Geometry check sheet. Reference: the model listing, model coordinates, mm. Face numbers are marked on the shaded views. A direction names the side the tool comes from. Coordinates: 2 decimals unless noted, no trailing zeros. Order: outer loops, then holes, each group sorted by start corner. A loop starts at its lowest first (then second) coordinate and runs counter-clockwise, first axis right, second up. Notation, with made-up numbers: M -24,71 L -1,71 A11 cw -1,79 Z; hole C 57.5,54 d2. An arc over 180 degrees is marked long. One line per item, written item: value. Start each with the question number.
1) Thickness scan on L1, parallel to Y at x = 0, z = 13.5; L2, parallel to X at y = 4, z = 17. Record the ranges inside material, lowest first. Write a range as from..to.
2) Go/stop test with flat-tipped pins: P1, Ø2.5, axis at x = 0, y = 0, coming from the -Z side; P2, Ø1.5, axis at x = 3.5, y = -1.5, coming from the -Z side; P3, Ø1.5, axis at y = -1.5, z = 31.5, coming from the -X side; P4, Ø3.5, axis at x = 0, y = 0, coming from the +Z side. Record where each tip stops, or that it passes through.
3) Sectioned sample at A-A, the plane x = 0. Enter the section's corners in (y, z).
4) Sectioned sample at D-D, the plane x = -3.5. Enter the section's corners in (y, z), then the cut area to 3 significant figures.
5) Draft check along Y on the marked faces 3, 4 and 5. Enter one of: pulls with the +Y half, pulls with the -Y half, needs draft (parallel to the pull), parting line crosses it, or undercut.
6) Sectioned sample at C-C, the plane z = 28. Enter the section's corners in (x, y), then the cut area to 3 significant figures.
7) Access from +Z, -Z, +X, -X, +Y, -Y to the whole of each face (thin tool, end or side, straight path). Record for the marked faces 1 and 2.
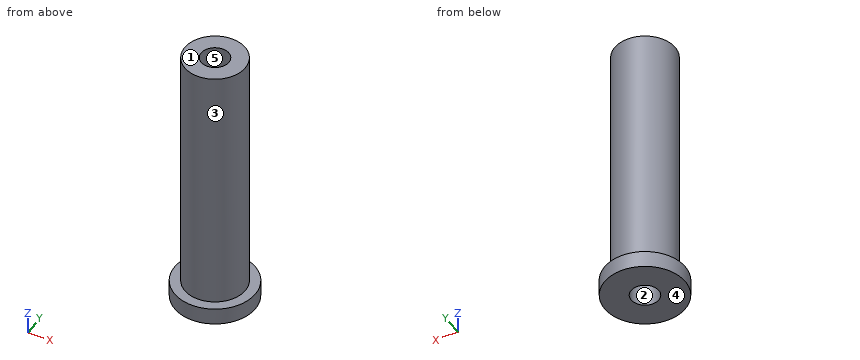
Solid Edge part; units mm, degrees
sketch "Sketch1" plane through (0, 0, 0) normal (0, 0, 1) x (1, 0, 0)
  circle A0 centre (0, 0) radius 4.5
extrude "Protrusion1" add sketch "Sketch1" along normal blind 40
sketch "Sketch2" plane through (0, 0, 0) normal (0, 0, 1) x (1, 0, 0)
  circle A0 centre (0, 0) radius 6
extrude "Extrusionsausprägung_2" add sketch "Sketch2" along normal blind 2.5
hole "Bohrung_3" at (0, 0, 0) direction (0, 0, 1) diameter 4.134 depth 15
hole "Bohrung_4" at (0, 0, 40) direction (0, 0, -1) diameter 4.134 depth 15
properties part number "21" material "Aluminiumlegierung:3.0205, Al 99.0, EN-AW 1200"
Final values:
1. L1: y = -4.5..-2.07, 2.07..4.5
1. L2: x = -2.06..2.06
2. P1: stops at z = 15
2. P2: stops at z = 0
2. P3: stops at x = -4.44
2. P4: stops at z = 25
3. outline: M -6,0 L -2.07,0 L -2.07,15 L 2.07,15 L 2.07,0 L 6,0 L 6,2.5 L 4.5,2.5 L 4.5,40 L 2.07,40 L 2.07,25 L -2.07,25 L -2.07,40 L -4.5,40 L -4.5,2.5 L -6,2.5 Z
4. outline: M -4.87,0 L 4.87,0 L 4.87,2.5 L 2.83,2.5 L 2.83,40 L -2.83,40 L -2.83,2.5 L -4.87,2.5 Z
4. area: 236 mm^2
5. face 3: parting line crosses it
5. face 4: needs draft
5. face 5: undercut
6. outline: C 0,0 d9; hole C 0,0 d4.13
6. area: 50.2 mm^2
7. face 1: +Z, +X, -X, +Y, -Y
7. face 2: -Z
